from build123d import *

# Parameters (mm, degrees)
ESQUISSE1_W                                        = 11
ESQUISSE1_H                                        = 6
BOSS_EXTRU_1_DEPTH                                 = 22
DIAM_TRE_DU_PER_AGE_7_1_7_1_1_D                    = 7.1
DIAM_TRE_DU_PER_AGE_7_1_7_1_1_DEPTH                = 6
DIAM_TRE_DU_PER_AGE_8_5_8_5_1_D                    = 8.5
CHAMBRAGE_POUR_VIS_T_TE_HEXAGONALE_M21_D           = 2.5
CHAMBRAGE_POUR_VIS_T_TE_HEXAGONALE_M21_CBORE_D     = 4
CHAMBRAGE_POUR_VIS_T_TE_HEXAGONALE_M21_CBORE_DEPTH = 4.5
DIAM_TRE_DU_PER_AGE_8_0_8_1_D                      = 8
DIAM_TRE_DU_PER_AGE_8_0_8_1_DEPTH                  = 2
DIAM_TRE_DU_PER_AGE_8_0_8_1_TIP                    = 4
CHANFREIN1_SIZE                                    = 9
CHANFREIN1_SIZE2                                   = 4.785384885


with BuildPart() as part:
    # Esquisse1 → Révolution1 (revolve)
    with BuildSketch(Plane(origin=(0, 0, 0), x_dir=(-1, 0, 0), z_dir=(0, 0, -1)), mode=Mode.PRIVATE) as r_volution1_sk:
        with Locations((-5.5, 3)):
            Rectangle(ESQUISSE1_W, ESQUISSE1_H)
    revolve(r_volution1_sk.sketch.rotate(Axis((0, 0, 0), (0, 1, 0)), 270), axis=Axis((0, 0, 0), (0, 1, 0)))

    # Esquisse2 → Boss.-Extru.1 (add)
    with BuildSketch(Plane(origin=(0, 6, 0), x_dir=(-1, 0, 0), z_dir=(0, 1, 0))):
        Polygon((-9.95156463, 2.63938656), (-3.016441782, 9.843834567), (10.088792211, -2.771484138), (3.016441782, -9.843834567), align=None)
    extrude(amount=BOSS_EXTRU_1_DEPTH)

    # Diamètre du perçage Ø7.1 (7.1)1
    with Locations(Plane(origin=(0, 28, 0), x_dir=(1, 0, 0), z_dir=(0, 1, 0))):
        with Locations((0, 0)):
            Hole(DIAM_TRE_DU_PER_AGE_7_1_7_1_1_D / 2, depth=DIAM_TRE_DU_PER_AGE_7_1_7_1_1_DEPTH)

    # Diamètre du perçage Ø8.5 (8.5)1 (through all)
    with Locations(Plane(origin=(-3.467561424, 0, 3.602224003), x_dir=(0.7204448006982934, 0, 0.6935122847843406), z_dir=(-0.6935122847843406, 0, 0.7204448006982934))):
        with Locations((-0.19047619, 17)):
            Hole(DIAM_TRE_DU_PER_AGE_8_5_8_5_1_D / 2)

    # Chambrage pour vis à tête hexagonale M21 (through all)
    with Locations(Plane(origin=(0, 6, 0), x_dir=(1, 0, 0), z_dir=(0, 1, 0))):
        with Locations((5.656854249, 5.656854249), (-5.656854249, -5.656854249)):
            CounterBoreHole(CHAMBRAGE_POUR_VIS_T_TE_HEXAGONALE_M21_D / 2, CHAMBRAGE_POUR_VIS_T_TE_HEXAGONALE_M21_CBORE_D / 2, CHAMBRAGE_POUR_VIS_T_TE_HEXAGONALE_M21_CBORE_DEPTH)

    # Diamètre du perçage Ø8.0 (8)1
    with Locations(Plane(origin=(0, 0, 0), x_dir=(-1, 0, 0), z_dir=(0, -1, 0))):
        with Locations((0, 0)):
            Hole(DIAM_TRE_DU_PER_AGE_8_0_8_1_D / 2, depth=DIAM_TRE_DU_PER_AGE_8_0_8_1_DEPTH)
            with Locations((0, 0, -(DIAM_TRE_DU_PER_AGE_8_0_8_1_DEPTH + DIAM_TRE_DU_PER_AGE_8_0_8_1_TIP / 2))):  # 90° drill point
                Cone(0, DIAM_TRE_DU_PER_AGE_8_0_8_1_D / 2, DIAM_TRE_DU_PER_AGE_8_0_8_1_TIP, mode=Mode.SUBTRACT)

    # Chanfrein1
    chanfrein1_edges = [part.edges().sort_by_distance(p)[0] for p in [
        (-6.552616997, 28, -6.307659352),
    ]]
    chanfrein1_side = [part.faces().sort_by_distance(p)[0] for p in [
        (-6.552616997, 17, -6.307659352),
    ]]
    chamfer(chanfrein1_edges, length=CHANFREIN1_SIZE, length2=CHANFREIN1_SIZE2, reference=chanfrein1_side[0])


solid = part.part
Design review of the part built by this model. Coordinates are the model's own, in mm. A direction names the side the tool comes from. Give positions to 0.01 mm unless a question says otherwise; leave off trailing zeros. Order: outer loops, then holes, each group sorted by start corner. A loop starts at its lowest first (then second) coordinate and runs counter-clockwise, first axis right, second up. Notation, with made-up numbers: (52.5, -23) - (108.5, -23) arc R32 ccw to (108.5, 3) - close; hole circle Ø5 at (54.5, 47). An arc over 180 degrees is marked (long way). Write item = value, one per line. Start each with the question number.
Q1. We need section C-C on z = -8.75. State the section outline as (x, y) points.
Q2. We need section A-A on y = 26.25. State the section outline as (x, z) points.
Q3. We need section B-B on x = -7.25. State the section outline as (y, z) points.
Q4. Tool access review of faces 5 (the face through (-7.131, 3.782, 4.305)), 6 (the face through (-0.53, 14.4, 6.43)), 7 (the face through (6.259, 14.402, -0.916)): name each direction out of +Z, -Z, +X, -X, +Y, -Y from which nothing blocks a thin tool from reaching the whole face with its end or side.
Q5. Mouldability with a two-part tool opening along Z and no side actions: class faces 1 (the face through (3.4, 28, 1.8)), 2 (the face through (0.575, 12.851, 0.456)), 3 (the face through (6.533, 16.846, 6.191)), 4 (the face through (-4.41, 0.74, 5.6)) as released by +Z, released by -Z, zero draft, split by the parting line, or undercut.
Q6. Clearance check with flat-ended pins moving along their axes: pin 1 Ø6 at (y, z) = (15, -8.5) entering from +X; pin 2 Ø4 at (x, z) = (8.5, -6.5) entering from +Y; pin 3 Ø3 at (y, z) = (24.5, -4.5) entering from +X. State where each tip first meets the part, or that it passes through.
Q7. We need section D-D on y = 9.25. State the section outline as (x, z) points, plus the area to 3 significant figures.
Q8. To check wall thickness, follow L1, parallel to Y at x = -3, z = 2.75; L2, parallel to Y at x = -5, z = 1.25; L3, parallel to Y at x = 7, z = -0.5. State the ranges of each line that lie inside material, in increasing order. Write a range as from..to.
Working result:
q1.outline = (-6.67, 0) - (6.67, 0) - (6.67, 6) - (-1.88, 6) - (-1.88, 21.97) - (-4.11, 19) - (-4.11, 6) - (-6.67, 6) - close
q2.outline = (-7.31, -0.1) - (-0.24, -7.17) - (9.95, 2.64) - (3.02, 9.84) - close; hole circle Ø7.1 at (0, 0)
q3.outline = (0, -8.27) - (6, -8.27) - (6, -5.61) - (19, -5.61) - (26.41, -0.04) - (6, -0.04) - (6, 4.45) - (1.5, 4.45) - (1.5, 6.87) - (6, 6.87) - (6, 8.27) - (0, 8.27) - close
q4.face_5 = +Y
q4.face_6 = +Z, -X, +Y
q4.face_7 = -Z, +X, +Y
q5.face_1 = zero draft
q5.face_2 = undercut
q5.face_3 = released by +Z
q5.face_4 = undercut
q6.pin_1 = 1.26
q6.pin_2 = 6
q6.pin_3 = 4.09
q7.outline = (-10.09, -2.77) - (-3.02, -9.84) - (9.95, 2.64) - (3.02, 9.84) - close
q7.area = 181 mm²
q8.L1 = 0..12.75, 21.25..28
q8.L2 = 0..13.6, 20.4..28
q8.L3 = 0..6
